from build123d import *

# Parameters (mm, degrees)
SKETCH1_W                                    = 5
SKETCH1_H                                    = 60
BOSS_EXTRUDE1_DEPTH                          = 57.5
M4_TAPPED_HOLE1_AT_2_COUNT                   = 2
M4_TAPPED_HOLE1_AT_2_PITCH                   = 107
M4_TAPPED_HOLE1_AT_3_COUNT                   = 2
M4_TAPPED_HOLE1_AT_3_PITCH                   = 49
M4_TAPPED_HOLE1_AT_4_COUNT                   = 2
M4_TAPPED_HOLE1_AT_4_PITCH                   = 117.686022959
CSK_FOR_M5_COUNTERSUNK_FLAT_HEAD_SCR_2_COUNT = 2
CSK_FOR_M5_COUNTERSUNK_FLAT_HEAD_SCR_2_PITCH = 77.956718761
CSK_FOR_M5_COUNTERSUNK_FLAT_HEAD_SCR_3_COUNT = 2
CSK_FOR_M5_COUNTERSUNK_FLAT_HEAD_SCR_3_PITCH = 67.5
CSK_FOR_M5_COUNTERSUNK_FLAT_HEAD_SCR_4_COUNT = 2
CSK_FOR_M5_COUNTERSUNK_FLAT_HEAD_SCR_4_PITCH = 39
FILLET1_R                                    = 0.5
CHAMFER1_SIZE                                = 0.5


with BuildPart() as part:
    # Sketch1 → Boss-Extrude1 (new body, symmetric)
    with BuildSketch(Plane(origin=(0, 0, 0), x_dir=(0, 0, -1), z_dir=(1, 0, 0))):
        Rectangle(SKETCH1_W, SKETCH1_H)
    extrude(amount=BOSS_EXTRUDE1_DEPTH, both=True)

    # Sketch3 → M4 Tapped Hole1 (revolve, cut)
    with BuildSketch(Plane(origin=(-53.5, 24.5, 2.5), x_dir=(0, -1, 0), z_dir=(1, 0, 0))):
        Polygon((0, 0), (0, 5), (2.025, 5), (1.65, 4.625), (1.65, 0.375), (2.025, 0), align=None)
    m4_tapped_hole1 = revolve(axis=Axis((-53.5, 24.5, 8.85), (0, 0, -1)), mode=Mode.SUBTRACT)

    # M4 Tapped Hole1 at 2: M4 Tapped Hole1 ×2
    with Locations(*[(i * M4_TAPPED_HOLE1_AT_2_PITCH, 0, 0) for i in range(1, M4_TAPPED_HOLE1_AT_2_COUNT)]):
        add(m4_tapped_hole1, mode=Mode.SUBTRACT)

    # M4 Tapped Hole1 at 3: M4 Tapped Hole1 ×2
    with Locations(*[(0, -i * M4_TAPPED_HOLE1_AT_3_PITCH, 0) for i in range(1, M4_TAPPED_HOLE1_AT_3_COUNT)]):
        add(m4_tapped_hole1, mode=Mode.SUBTRACT)

    # M4 Tapped Hole1 at 4: M4 Tapped Hole1 ×2
    with Locations(*[Vector(0.909198878, -0.416362103, 0) * (i * M4_TAPPED_HOLE1_AT_4_PITCH) for i in range(1, M4_TAPPED_HOLE1_AT_4_COUNT)]):
        add(m4_tapped_hole1, mode=Mode.SUBTRACT)

    # Sketch6 → CSK for M5 Countersunk Flat Head Screw1 (revolve, cut)
    with BuildSketch(Plane(origin=(-22, 19.5, -2.5), x_dir=(0, 1, 0), z_dir=(1, 0, 0))):
        Polygon((0, 0), (0, 5), (2.775, 5), (2.75, 4.975), (2.75, 3.45), (5.2, 1), (5.2, 0), align=None)
    csk_for_m5_countersunk_flat_head_screw1 = revolve(axis=Axis((-22, 19.5, -8.85), (0, 0, 1)), mode=Mode.SUBTRACT)

    # CSK for M5 Countersunk Flat Head Scr 2: CSK for M5 Countersunk Flat Head Screw1 ×2
    with Locations(*[Vector(0.865865073, -0.500277598, 0) * (i * CSK_FOR_M5_COUNTERSUNK_FLAT_HEAD_SCR_2_PITCH) for i in range(1, CSK_FOR_M5_COUNTERSUNK_FLAT_HEAD_SCR_2_COUNT)]):
        add(csk_for_m5_countersunk_flat_head_screw1, mode=Mode.SUBTRACT)

    # CSK for M5 Countersunk Flat Head Scr 3: CSK for M5 Countersunk Flat Head Screw1 ×2
    with Locations(*[(i * CSK_FOR_M5_COUNTERSUNK_FLAT_HEAD_SCR_3_PITCH, 0, 0) for i in range(1, CSK_FOR_M5_COUNTERSUNK_FLAT_HEAD_SCR_3_COUNT)]):
        add(csk_for_m5_countersunk_flat_head_screw1, mode=Mode.SUBTRACT)

    # CSK for M5 Countersunk Flat Head Scr 4: CSK for M5 Countersunk Flat Head Screw1 ×2
    with Locations(*[(0, -i * CSK_FOR_M5_COUNTERSUNK_FLAT_HEAD_SCR_4_PITCH, 0) for i in range(1, CSK_FOR_M5_COUNTERSUNK_FLAT_HEAD_SCR_4_COUNT)]):
        add(csk_for_m5_countersunk_flat_head_screw1, mode=Mode.SUBTRACT)

    # Fillet1
    fillet1_edges = [part.edges().sort_by_distance(p)[0] for p in [
        (0, -30, -2.5),
        (0, -30, 2.5),
        (0, 30, 2.5),
        (0, 30, -2.5),
    ]]
    fillet(fillet1_edges, radius=FILLET1_R)

    # Chamfer1
    chamfer1_edges = [part.edges().sort_by_distance(p)[0] for p in [
        (-57.5, 0, -2.5),
        (57.5, 0, -2.5),
        (-57.5, -30, 0),
        (-57.5, 0, 2.5),
        (-57.5, 30, 0),
        (-57.5, 29.853553391, 2.353553391),
        (-57.5, 29.853553391, -2.353553391),
        (-57.5, -29.853553391, 2.353553391),
        (-57.5, -29.853553391, -2.353553391),
        (57.5, -30, 0),
        (57.5, 30, 0),
        (57.5, 0, 2.5),
        (57.5, 29.853553391, 2.353553391),
        (57.5, 29.853553391, -2.353553391),
        (57.5, -29.853553391, 2.353553391),
        (57.5, -29.853553391, -2.353553391),
    ]]
    chamfer(chamfer1_edges, length=CHAMFER1_SIZE)


solid = part.part
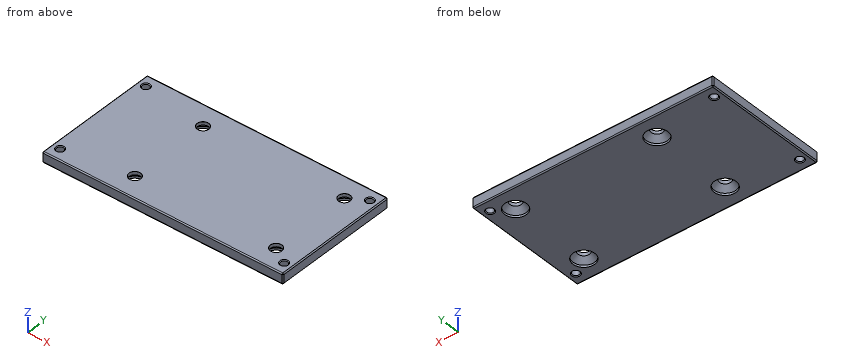
The listing builds one solid part. Answer for the finished solid, in the listing's coordinates (mm). Give positions to 0.01 mm unless a question says otherwise; leave off trailing zeros. Write each loop counter-clockwise with the first axis right and the second up, starting at its lowest first coordinate (ties: lowest second). Pieces come first, ordered by that corner, then holes. Notation, with made-up numbers: (-21.5, 63) -> (31.5, 63) arc R20 ccw to (31.5, 95) -> close; hole circle Ø1 at (23.25, 61). An arc over 180 degrees is marked (long way). One line per question, with ' | ' between items. Start each with the question number.
1. Given pin 1 Ø4 at (x, y) = (53.5, 24.5) entering from +Z (3 decimals); pin 2 Ø9 at (x, y) = (-22, -19.5) entering from -Z, each flat-ended and moving along its own axis, determine where each tip first touches the part or whether it passes through.
2. Section A-A (x = 53.5) is taken. Determine the outline of the cut face in (y, z) (3 decimals).
3. Section C-C (z = -0.3) is taken. State how many separate pieces and enclosed holes the cut face has, plus the area to 3 significant figures.
4. Section B-B (y = -19.5) is taken. Determine the outline of the cut face in (x, z) (3 decimals).
5. Find the intervals of material crossed by probe 1 along Y at (x, z) = (-22, -1.75); probe 2 along X at (y, z) = (-19.5, -1.9); probe 3 along Y at (x, z) = (-53.5, -0.45), in increasing order.
Response values:
1) pin 1: z = 2.475 | pin 2: z = -0.8
2) outline: (-30, -2) arc R0.5 ccw to (-29.5, -2.5) -> (-26.525, -2.5) -> (-26.15, -2.125) -> (-26.15, 2.125) -> (-26.525, 2.5) -> (-29.5, 2.5) arc R0.5 ccw to (-30, 2) -> close; (-22.85, -2.125) -> (-22.475, -2.5) -> (22.475, -2.5) -> (22.85, -2.125) -> (22.85, 2.125) -> (22.475, 2.5) -> (-22.475, 2.5) -> (-22.85, 2.125) -> close; (26.15, -2.125) -> (26.525, -2.5) -> (29.5, -2.5) arc R0.5 ccw to (30, -2) -> (30, 2) arc R0.5 ccw to (29.5, 2.5) -> (26.525, 2.5) -> (26.15, 2.125) -> close
3) separate pieces: 1 | enclosed holes: 8 | area: 6,660 mm2
4) outline: (-57.5, -2) -> (-57, -2.5) -> (-27.2, -2.5) -> (-27.2, -1.5) -> (-24.75, 0.95) -> (-24.75, 2.475) -> (-24.775, 2.5) -> (-57, 2.5) -> (-57.5, 2) -> close; (-19.25, 0.95) -> (-16.8, -1.5) -> (-16.8, -2.5) -> (40.3, -2.5) -> (40.3, -1.5) -> (42.75, 0.95) -> (42.75, 2.475) -> (42.725, 2.5) -> (-19.225, 2.5) -> (-19.25, 2.475) -> close; (48.25, 0.95) -> (50.7, -1.5) -> (50.7, -2.5) -> (57, -2.5) -> (57.5, -2) -> (57.5, 2) -> (57, 2.5) -> (48.275, 2.5) -> (48.25, 2.475) -> close
5) probe 1: -30 to -24.7, -14.3 to 14.3, 24.7 to 30 | probe 2: -57.5 to -27.2, -16.8 to 40.3, 50.7 to 57.5 | probe 3: -30 to -26.15, -22.85 to 22.85, 26.15 to 30
